Check sheet for the modelled part. Datum: model origin and axes. Units: mm. Coordinates: 2 decimals unless noted, no trailing zeros. Write each loop counter-clockwise with the first axis right and the second up, starting at its lowest first coordinate (ties: lowest second). Pieces come first, ordered by that corner, then holes. Notation, with made-up numbers: M 80.5,11 L 86.5,11 A25 cw 86.5,47 Z; hole C -38,73 d4. An arc over 180 degrees is marked long. Answer as CSV lines item,"result". Start each with the question number.
Q1. Thickness scan on line 1 along X through (y, z) = (-0.25, 0.55); line 2 along X through (y, z) = (-0.5, 0.4); line 3 along Y through (x, z) = (0, 0.55). Record the ranges inside material, lowest first. Write a range as from..to.
Q2. Sectioned sample at C-C, the plane z = 0.5. Record the cut outline in (x, y).
Q3. Sectioned sample at A-A, the plane x = 0. Record the cut outline in (y, z).
Q4. Sectioned sample at D-D, the plane y = -2.25. Record the cut outline in (x, z), then the cut area to 3 significant figures.
Q5. Mould release check, pull along X, two halves, no side actions. Record for faces 1 (the cylindrical face through (-0.867, 3.905, 0.493)), 2 (the flat face through (2, -1, 1)), 3 (the cylindrical face through (-0.07, 1.5, 0.35)): pulls with the +X half, pulls with the -X half, needs draft (parallel to the pull), parting line crosses it, or undercut.
Autodesk Inventor part; units mm, degrees
ref_plane "YZ Plane" through (0, 0, 0) normal (1, 0, 0) x (0, 1, 0)
ref_plane "XZ Plane" through (0, 0, 0) normal (0, 1, 0) x (-1, 0, 0)
ref_plane "XY Plane" through (0, 0, 0) normal (0, 0, 1) x (1, 0, 0)
sketch "スケッチ1" plane through (0, 0, 0) normal (0, 0, 1) x (1, 0, 0)
  circle A0 centre (0, 0) radius 4
  dimension "d0" = 8
extrude "押し出し1" add sketch "スケッチ1" along normal blind 1
sketch "スケッチ2" plane through (0, 0, 1) normal (0, 0, 1) x (1, 0, 0)
  circle A0 centre (0, 0) radius 1.5
  dimension "d3" = 3
hole "穴1" at (0, 0, 1) direction (0, 0, -1) diameter 3 end through all
chamfer "面取り1" distance 0.3 angle 45 1 edges at (0, 1.5, 1)
properties part number "RD019_ブッシュ80F-0305改"
Output:
1,line 1,"x = -3.99..-1.48, 1.48..3.99"
1,line 2,"x = -3.97..-1.41, 1.41..3.97"
1,line 3,"y = -4..-1.5, 1.5..4"
2,outline,"C 0,0 d8; hole C 0,0 d3"
3,outline,"M -4,0 L -1.5,0 L -1.5,0.7 L -1.8,1 L -4,1 Z; M 1.5,0 L 4,0 L 4,1 L 1.8,1 L 1.5,0.7 Z"
4,outline,"M -3.31,0 L 3.31,0 L 3.31,1 L -3.31,1 Z"
4,area,"6.61 mm^2"
5,face 1,"parting line crosses it"
5,face 2,"needs draft"
5,face 3,"undercut"
